The listing builds one solid part. Answer for the finished solid, in the listing's coordinates (mm). Face numbers are marked on the shaded views. A direction names the side the tool comes from. Round coordinates to 2 decimals unless told otherwise and drop trailing zeros. Write each loop counter-clockwise with the first axis right and the second up, starting at its lowest first coordinate (ties: lowest second). Pieces come first, ordered by that corner, then holes. Notation, with made-up numbers: (39, 79) - (56, 79) arc R17 ccw to (56, 92) - close; hole circle Ø1 at (6.25, 5). An arc over 180 degrees is marked (long way). Return JSON: item names as keys, results as strings. Group by question number.
(1) Which of the six approach directions +Z, -Z, +X, -X, +Y, -Y give full straight-line access (tool end or side, diameter ignored) to the marked faces 5 and 6?
(2) Section C-C, the plane z = 4.25 is taken. Write down the section's boundary in (x, y), then the cut area to 3 significant figures.
(3) Determine the mould class of the marked faces 1, 2, 3 and 4 for opening direction Y: +Y half, -Y half, draft (parallel to the pull), parting line (faces both ways), or undercut.
(4) Section A-A, the plane y = -0.5 is taken. Write down the section's boundary in (x, z), then the cut area to 3 significant figures.
(5) Section B-B, the plane x = 0 is taken. Write down the section's boundary in (y, z).
(6) Section D-D, the plane x = -6 is taken. Write down the section's boundary in (y, z).
(7) Find the intervals of material crossed by line 1 along Y through (x, z) = (0, 2.5); line 2 along Y through (x, z) = (0, 6.75); line 3 along Z through (x, y) = (-8.75, -7.5), in increasing order. Write a range as [from, to].
(8) This flat-tipped pin is pushed along its axis until it touches: pin 1 (2 mm diameter, centred on x = -3, y = 7.5, fed in from +Z). Where does it stop, or does it pass through?
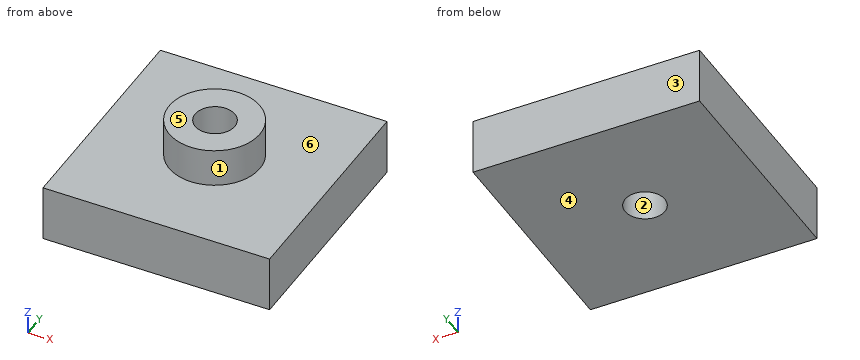
```python
from build123d import *

# Parameters (mm, degrees)
SKETCH_W     = 20
SKETCH_H     = 20
PAD_DEPTH    = 5
SKETCH001_R  = 4
PAD001_DEPTH = 3.4
SKETCH002_R  = 1.75
POCKET_DEPTH = 8.401


with BuildPart() as part:
    # Sketch → Pad (new body)
    with BuildSketch(Plane.XY):
        Rectangle(SKETCH_W, SKETCH_H)
    extrude(amount=PAD_DEPTH)

    # Sketch001 → Pad001 (new body)
    with BuildSketch(Plane.XY.offset(5)):
        with Locations((-0.047954, 0.023977)):
            Circle(SKETCH001_R)
    extrude(amount=PAD001_DEPTH)

    # Sketch002 → Pocket (cut, through all)
    with BuildSketch(Plane.XY.offset(8.4)):
        Circle(SKETCH002_R)
    extrude(amount=-POCKET_DEPTH, mode=Mode.SUBTRACT)


solid = part.part
```
Working result:
{
 "1": {"face 5": "+Z, +X, -X, +Y, -Y", "face 6": "+Z"},
 "2": {"outline": "(-10, -10) - (10, -10) - (10, 10) - (-10, 10) - close; hole circle Ø3.5 at (0, 0)", "area": "390 mm^2"},
 "3": {"face 1": "parting line", "face 2": "undercut", "face 3": "+Y half", "face 4": "draft"},
 "4": {"outline": "(-10, 0) - (-1.68, 0) - (-1.68, 8.4) - (-4.01, 8.4) - (-4.01, 5) - (-10, 5) - close; (1.68, 0) - (10, 0) - (10, 5) - (3.92, 5) - (3.92, 8.4) - (1.68, 8.4) - close", "area": "98.8 mm^2"},
 "5": {"outline": "(-10, 0) - (-1.75, 0) - (-1.75, 8.4) - (-3.98, 8.4) - (-3.98, 5) - (-10, 5) - close; (1.75, 0) - (10, 0) - (10, 5) - (4.02, 5) - (4.02, 8.4) - (1.75, 8.4) - close"},
 "6": {"outline": "(-10, 0) - (10, 0) - (10, 5) - (-10, 5) - close"},
 "7": {"line 1": "y = [-10, -1.75], [1.75, 10]", "line 2": "y = [-3.98, -1.75], [1.75, 4.02]", "line 3": "z = [0, 5]"},
 "8": {"pin 1": "stops at z = 5"}
}
